Geometry: see drawing. Coordinates: mm, zero at the bounding-box minimum. Give positions to 0.01 mm unless a question says otherwise; leave off trailing zeros. Loops run counter-clockwise (first coordinate to the right, second up) from the corner with the lowest first, then second, coordinate; pieces in that order, holes last. Notation, with made-up numbers: M -27.5,-3.75 L 12.5,-3.75 A10 ccw 12.5,0.25 Z; hole C 66.25,75.25 d11. An arc over 180 degrees is marked long. Use a Markdown table: item, result. Add a question column.
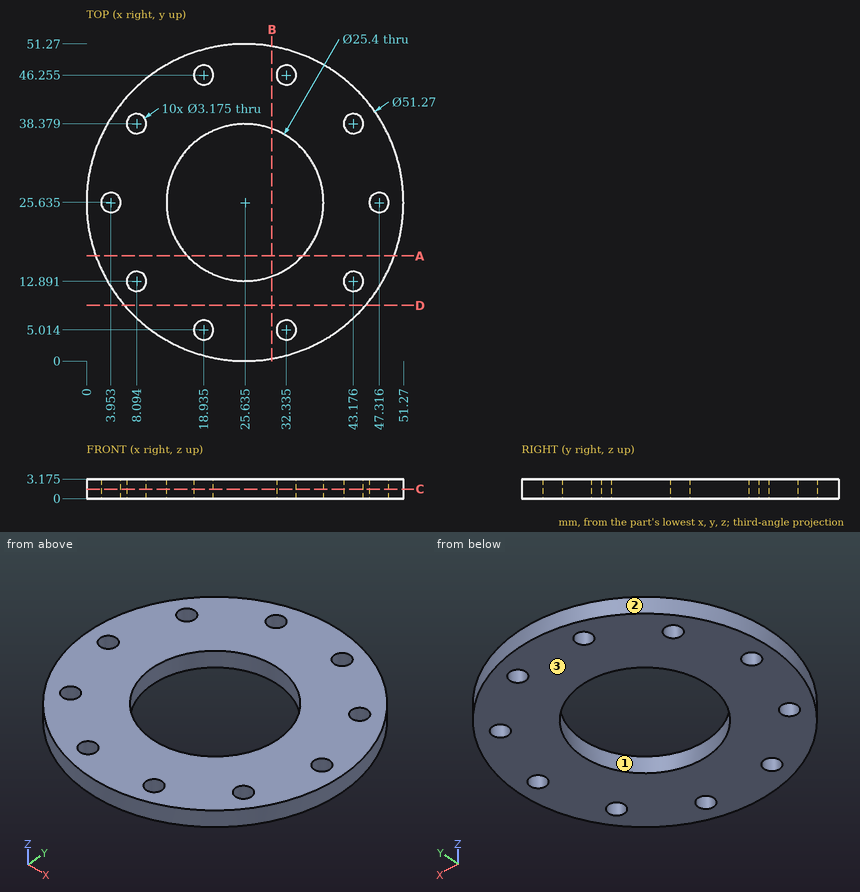
1) Section query B-B, the plane x = 30. Return the cut outline in (y, z) (1 decimal).
2) Pull-direction query (Y, two-part tool) for the marked faces 1, 2 and 3; classes: pulls with the +Y half, pulls with the -Y half, needs draft (parallel to the pull), parting line crosses it, or undercut.
3) Ray query, line 1 (Y direction, x = 8, z = 3) (1 decimal); line 2 (X direction, y = 27, z = 2.3) (1 decimal); line 3 (Y direction, x = 33, z = 2.8) (1 decimal). Return the intervals inside material, ascending. Write a range as [from, to].
4) Section query C-C, the plane z = 1.55. State how many separate pieces and enclosed holes the cut face has, and give its area (3 significant figures).
5) Contact query for flat-ended pins moving along their axis: P1, Ø3, axis at x = 18.93, y = 5.01, coming from the +Z side; P2, Ø1.5, axis at y = 18, z = 1, coming from the +X side; P3, Ø1, axis at y = 35.5, z = 0.5, coming from the -X side. Output: stop coordinate, or through.
6) Section query D-D, the plane y = 9. Return the cut outline in (x, z) (1 decimal).
7) Section query A-A, the plane y = 17. Return the cut outline in (x, z) (1 decimal).
Entries:
| question | item | result |
|---|---|---|
| 1 | outline | M 0.4,0 L 13.7,0 L 13.7,3.2 L 0.4,3.2 Z; M 37.6,0 L 50.9,0 L 50.9,3.2 L 37.6,3.2 Z |
| 2 | face 1 | undercut |
| 2 | face 2 | parting line crosses it |
| 2 | face 3 | needs draft |
| 3 | line 1 | y = [7, 11.3], [14.5, 36.8], [40, 44.2] |
| 3 | line 2 | x = [0, 3.1], [4.8, 13], [38.3, 46.5], [48.1, 51.2] |
| 3 | line 3 | y = [1.1, 3.6], [6.5, 15.3], [36, 44.8], [47.7, 50.2] |
| 4 | separate pieces | 1 |
| 4 | enclosed holes | 11 |
| 4 | area | 1,480 mm² |
| 5 | P1 | passes through |
| 5 | P2 | stops at x = 50.33 |
| 5 | P3 | stops at x = 1.77 |
| 6 | outline | M 6.1,0 L 45.1,0 L 45.1,3.2 L 6.1,3.2 Z |
| 7 | outline | M 1.5,0 L 16.3,0 L 16.3,3.2 L 1.5,3.2 Z; M 34.9,0 L 49.8,0 L 49.8,3.2 L 34.9,3.2 Z |
